The drawing under review shows one solid part. Ordinate dimensions are in mm from its lowest x, y, z. A direction names the side the tool comes from. Give positions to 0.01 mm unless a question says otherwise; leave off trailing zeros. Loops run counter-clockwise (first coordinate to the right, second up) from the corner with the lowest first, then second, coordinate; pieces in that order, holes last.
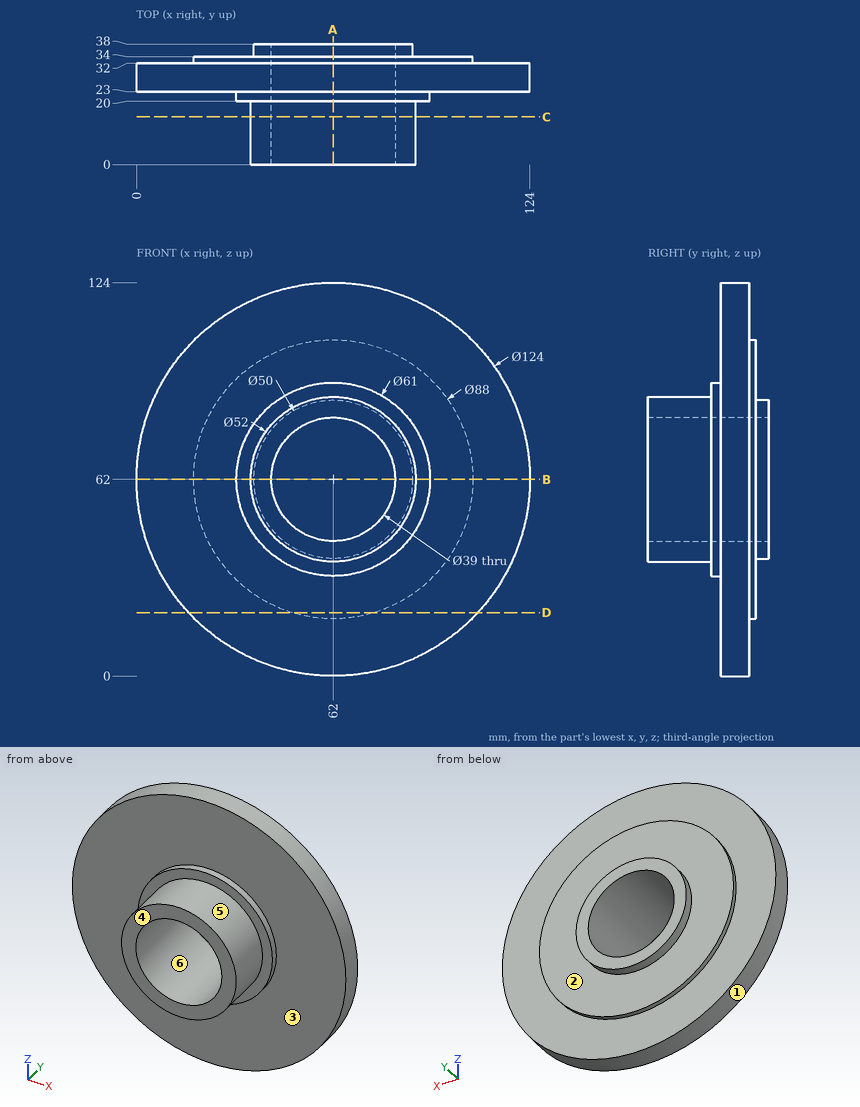
Item 1: Take a section at B-B on z = 62. Give the boundary of the cut face in (x, y), and give its area (3 significant figures).
Answer:
outline: (0, 23) - (31.5, 23) - (31.5, 20) - (36, 20) - (36, 0) - (42.5, 0) - (42.5, 38) - (37, 38) - (37, 34) - (18, 34) - (18, 32) - (0, 32) - close; (81.5, 0) - (88, 0) - (88, 20) - (92.5, 20) - (92.5, 23) - (124, 23) - (124, 32) - (106, 32) - (106, 34) - (87, 34) - (87, 38) - (81.5, 38) - close
area: 1,230 mm2
Item 2: For L1, parallel to Z at x = 62, y = 13; L2, parallel to Z at x = 62, y = 22; L3, parallel to Y at x = 83, z = 41.5, list the stretches that pass through material, from the lowest coordinate up.
Answer:
L1: z = 36 to 42.5, 81.5 to 88
L2: z = 31.5 to 42.5, 81.5 to 92.5
L3: y = 20 to 34
Item 3: Take a section at C-C on y = 15. Give the boundary of the cut face in (x, z).
Answer:
outline: circle Ø52 at (62, 62); hole circle Ø39 at (62, 62)
Item 4: Tool access review of the marked faces 1, 2 and 3: name each direction out of +Z, -Z, +X, -X, +Y, -Y from which nothing blocks a thin tool from reaching the whole face with its end or side.
Answer:
face 1: +Y, -Y
face 2: +Y
face 3: -Y
Item 5: The part is to be moulded in two halves that separate along X. For the marked faces 4, 5 and 6, say which applies: released by +X, released by -X, zero draft, split by the parting line, or undercut.
Answer:
face 4: zero draft
face 5: split by the parting line
face 6: undercut
Item 6: Clearance check with flat-ended pins moving along their axes: pin 1 Ø12 at (y, z) = (26, 95.5) entering from -X; pin 2 Ø12 at (x, y) = (61.5, 34) entering from +Z; pin 3 Ø10 at (x, z) = (88, 109.5) entering from -Y. State where each tip first meets the part, or that it passes through.
Answer:
pin 1: stops at x = 6.43
pin 2: stops at z = 124
pin 3: stops at y = 23
Item 7: Take a section at A-A on x = 62. Give the boundary of the cut face in (y, z).
Answer:
outline: (0, 36) - (20, 36) - (20, 31.5) - (23, 31.5) - (23, 0) - (32, 0) - (32, 18) - (34, 18) - (34, 37) - (38, 37) - (38, 42.5) - (0, 42.5) - close; (0, 81.5) - (38, 81.5) - (38, 87) - (34, 87) - (34, 106) - (32, 106) - (32, 124) - (23, 124) - (23, 92.5) - (20, 92.5) - (20, 88) - (0, 88) - close
Item 8: Take a section at D-D on z = 20. Give the boundary of the cut face in (x, y), and give its area (3 significant figures).
Answer:
outline: (16.39, 23) - (107.61, 23) - (107.61, 32) - (75.11, 32) - (75.11, 34) - (48.89, 34) - (48.89, 32) - (16.39, 32) - close
area: 873 mm2
